Part print with two shaded views. Sizes in mm from the minimum x, y, z corner. A direction names the side the tool comes from. Coordinates: 2 decimals unless noted, no trailing zeros. Order: outer loops, then holes, each group sorted by start corner. A loop starts at its lowest first (then second) coordinate and runs counter-clockwise, first axis right, second up.
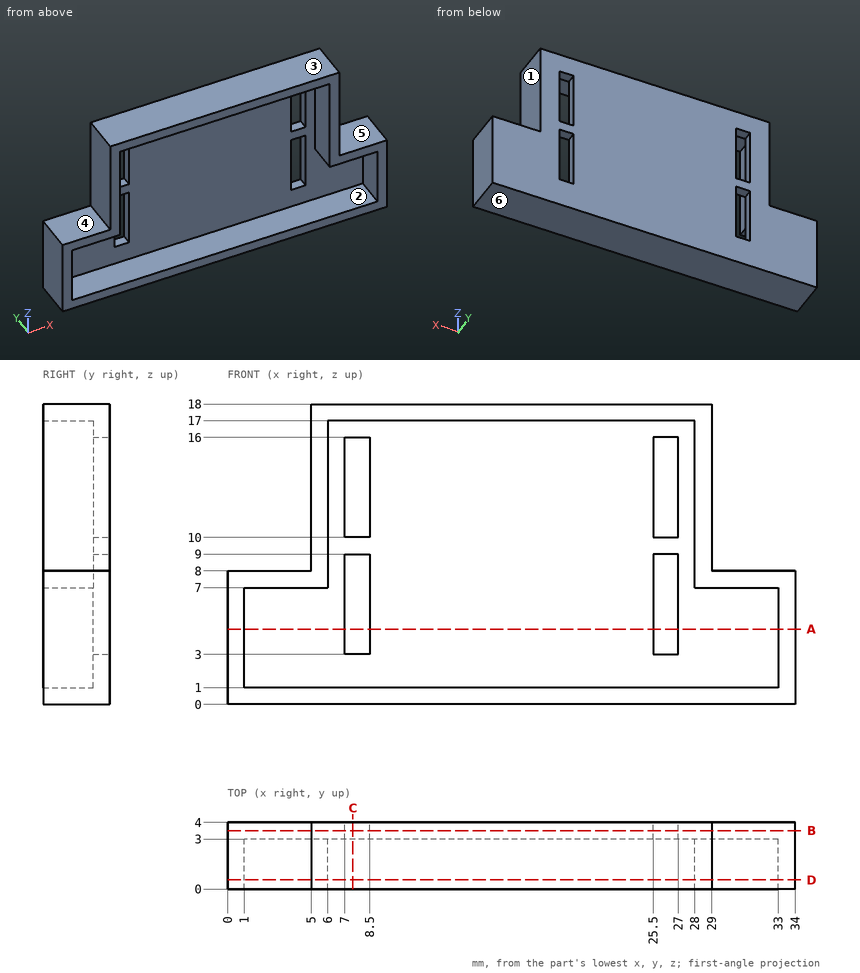
Q1. Cut at C-C on x = 7.5. Write the cut outline in (y, z).
Results list:
outline: (0, 0) - (4, 0) - (4, 3) - (3, 3) - (3, 1) - (0, 1) - close; (0, 17) - (3, 17) - (3, 16) - (4, 16) - (4, 18) - (0, 18) - close; (3, 9) - (4, 9) - (4, 10) - (3, 10) - close
Q2. Which spindle directions (+Z, -Z, +X, -X, +Y, -Y) get a long thin tool onto all of the face, cutting with end or side? Do the marked faces 4, 5 and 6. Say none if no direction does.
Results list:
face 4: +Z, -X, +Y, -Y
face 5: +Z, +X, +Y, -Y
face 6: -Z, +X, -X, +Y, -Y
Q3. Mould opens along Z. For the marked faces 1, 2 and 3 say: pulls with the +Z half, pulls with the -Z half, needs draft (parallel to the pull), parting line crosses it, or undercut.
Results list:
face 1: needs draft
face 2: undercut
face 3: pulls with the +Z half
Q4. Wall check: line 1 along X through (y, z) = (3.65, 13.25); line 2 along Z through (x, y) = (4.5, 1); line 3 along Z through (x, y) = (18, 1.6). Give the ranges that are in metal, low to high.
Results list:
line 1: x = 5 to 7, 8.5 to 25.5, 27 to 29
line 2: z = 0 to 1, 7 to 8
line 3: z = 0 to 1, 17 to 18
Q5. Cut at D-D on y = 0.55. Write the cut outline in (x, z), and give its area (3 significant figures).
Results list:
outline: (0, 0) - (34, 0) - (34, 8) - (29, 8) - (29, 18) - (5, 18) - (5, 8) - (0, 8) - close; hole (1, 1) - (33, 1) - (33, 7) - (28, 7) - (28, 17) - (6, 17) - (6, 7) - (1, 7) - close
area: 100 mm2
Q6. Cut at A-A on z = 4.5. Write the cut outline in (x, y), and give its area (3 significant figures).
Results list:
outline: (0, 0) - (1, 0) - (1, 3) - (7, 3) - (7, 4) - (0, 4) - close; (8.5, 3) - (25.5, 3) - (25.5, 4) - (8.5, 4) - close; (27, 3) - (33, 3) - (33, 0) - (34, 0) - (34, 4) - (27, 4) - close
area: 37.0 mm2
Q7. Cut at B-B on y = 3.5. Write the cut outline in (x, z).
Results list:
outline: (0, 0) - (34, 0) - (34, 8) - (29, 8) - (29, 18) - (5, 18) - (5, 8) - (0, 8) - close; hole (7, 3) - (8.5, 3) - (8.5, 9) - (7, 9) - close; hole (7, 10) - (8.5, 10) - (8.5, 16) - (7, 16) - close; hole (25.5, 3) - (27, 3) - (27, 9) - (25.5, 9) - close; hole (25.5, 10) - (27, 10) - (27, 16) - (25.5, 16) - close
Q8. Pin check, flat tips, straight feed: pin 1 Ø2 at (x, y) = (1.5, 3) entering from +Z; pin 2 Ø0.8 at (y, z) = (3.5, 13.5) entering from -X. Stop position of each tip, or through.
Results list:
pin 1: stops at z = 8
pin 2: stops at x = 5
